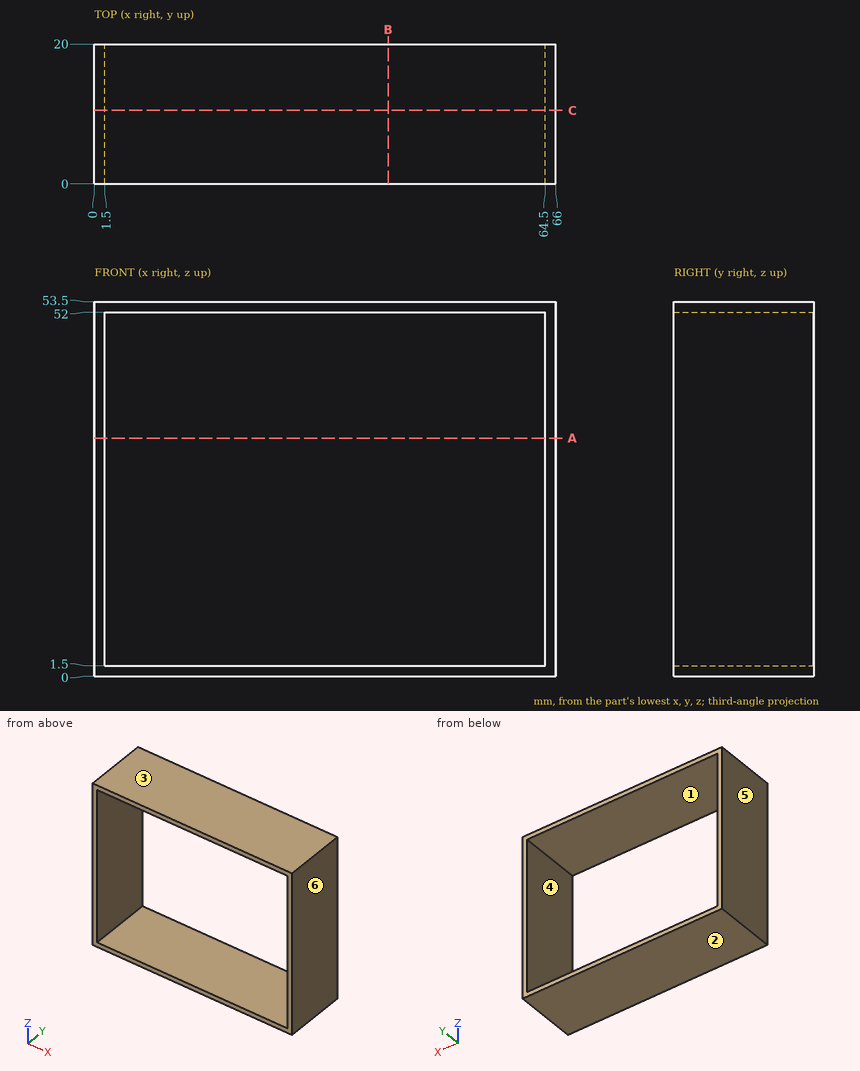
Job drawing, mm, ordinate dimensions from the low corner. One solid piece. A direction names the side the tool comes from. Round coordinates to 2 decimals unless told otherwise and drop trailing zeros. Write each loop counter-clockwise with the first axis right and the second up, starting at its lowest first coordinate (ties: lowest second). Pieces come first, ordered by that corner, then holes. Notation, with made-up numbers: (46, -28.5) -> (105, -28.5) arc R19 cw to (105, 3.5) -> close; hole circle Ø9 at (65.5, 42.5). An arc over 180 degrees is marked (long way). Answer as a JSON object with one key per item and string values.
(1) Which spindle directions (+Z, -Z, +X, -X, +Y, -Y) get a long thin tool onto all of the face, cutting with end or side? Do the marked faces 1 and 2. Say none if no direction does.
Reported:
{"face 1": "+Y, -Y", "face 2": "-Z, +X, -X, +Y, -Y"}
(2) Two-plate mould, pull along X, no slides. Class the marked faces 3, 4, 5 and 6: +X half, -X half, draft (parallel to the pull), parting line (faces both ways), or undercut.
Reported:
{"face 3": "draft", "face 4": "undercut", "face 5": "-X half", "face 6": "+X half"}
(3) Band-saw the part on A-A, the plane z = 34. List the corners of the cut face in (x, y), then the cut area to 3 significant figures.
Reported:
{"outline": "(0, 0) -> (1.5, 0) -> (1.5, 20) -> (0, 20) -> close; (64.5, 0) -> (66, 0) -> (66, 20) -> (64.5, 20) -> close", "area": "60.0 mm^2"}
(4) Band-saw the part on B-B, the plane x = 42. List the corners of the cut face in (y, z), then the cut area to 3 significant figures.
Reported:
{"outline": "(0, 0) -> (20, 0) -> (20, 1.5) -> (0, 1.5) -> close; (0, 52) -> (20, 52) -> (20, 53.5) -> (0, 53.5) -> close", "area": "60.0 mm^2"}
(5) Probe probe 1 along Z at (x, y) = (28, 12.75); probe 2 along X at (y, z) = (11.5, 37.5). List the from-to ranges inside material, lowest first. Write a range as [from, to].
Reported:
{"probe 1": "z = [0, 1.5], [52, 53.5]", "probe 2": "x = [0, 1.5], [64.5, 66]"}
(6) Band-saw the part on C-C, the plane y = 10.5. List the corners of the cut face in (x, z), then the cut area to 4 significant figures.
Reported:
{"outline": "(0, 0) -> (66, 0) -> (66, 53.5) -> (0, 53.5) -> close; hole (1.5, 1.5) -> (64.5, 1.5) -> (64.5, 52) -> (1.5, 52) -> close", "area": "349.5 mm^2"}
